Geometry check sheet. Reference: the model listing, model coordinates, mm. Face numbers are marked on the shaded views. A direction names the side the tool comes from. Give positions to 0.01 mm unless a question says otherwise; leave off trailing zeros. Write each loop counter-clockwise with the first axis right and the second up, starting at its lowest first coordinate (ties: lowest second). Pieces come first, ordered by that corner, then holes. Notation, with made-up numbers: (-2.75, 82.5) -> (21.25, 82.5) arc R11 cw to (21.25, 92.5) -> close; hole circle Ø5 at (-2, 31). An arc over 180 degrees is marked (long way). Write item = value, one per line. Start each with the question number.
1. Mould release check, pull along Y, two halves, no side actions. Record for the marked faces 1, 2 and 3: pulls with the +Y half, pulls with the -Y half, needs draft (parallel to the pull), parting line crosses it, or undercut.
2. Cross-section at A-A, the plane y = 21.5. Record the cut outline in (x, z), plus the area to 3 significant figures.
3. Cross-section at C-C, the plane x = -64. Record the cut outline in (y, z), plus the area to 3 significant figures.
4. Thickness scan on line 1 along X through (y, z) = (-19, 72); line 2 along Z through (x, y) = (-45.5, -22). Record the ranges inside material, lowest first.
5. Cross-section at B-B, the plane z = 35. Record the cut outline in (x, y).
6. Depth check by flat-ended pin: P1, Ø1.5, axis at x = -28.5, y = -27, coming from the +Z side; P2, Ø3, axis at y = 12.5, z = 93, coming from the -X side. Enter the tip coordinate at first touch or a pass-through.
7. Set-up check for the marked faces 4 and 5: record each of +Z, -Z, +X, -X, +Y, -Y from which the full face is reachable in a straight line by a thin tool's end or side.
```python
from build123d import *

# Parameters (mm, degrees)
F1_DEPTH      = 38.1
F1_DEPTH_BACK = 38.1


with BuildPart() as f1:
    # F0 (on Front) → F1 (new body, two sides)
    with BuildSketch(Plane.XZ) as f1_sk:
        Polygon((0, 0), (0, 152.4), (-25.4, 152.4), (-25.4, 25.4), (-76.2, 25.4), (-76.2, 0), align=None)
    extrude(amount=F1_DEPTH)
    extrude(f1_sk.sketch, amount=-F1_DEPTH_BACK)


solid = f1.part
```
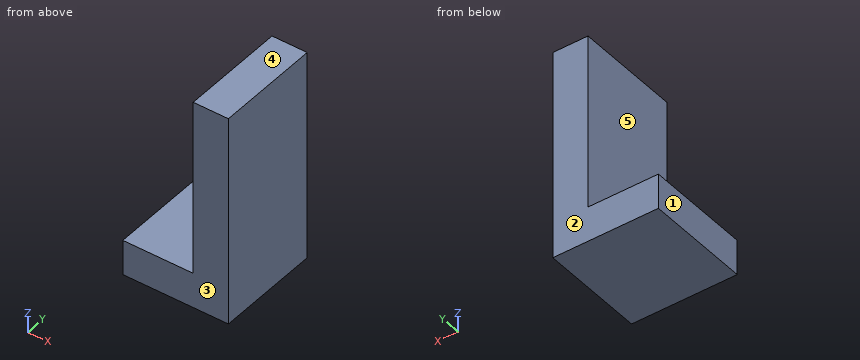
Answers:
q1.face_1 = needs draft
q1.face_2 = pulls with the +Y half
q1.face_3 = pulls with the -Y half
q2.outline = (-76.2, 0) -> (0, 0) -> (0, 152.4) -> (-25.4, 152.4) -> (-25.4, 25.4) -> (-76.2, 25.4) -> close
q2.area = 5,160 mm^2
q3.outline = (-38.1, 0) -> (38.1, 0) -> (38.1, 25.4) -> (-38.1, 25.4) -> close
q3.area = 1,940 mm^2
q4.line_1 = -25.4 to 0
q4.line_2 = 0 to 25.4
q5.outline = (-25.4, -38.1) -> (0, -38.1) -> (0, 38.1) -> (-25.4, 38.1) -> close
q6.P1 = 25.4
q6.P2 = -25.4
q7.face_4 = +Z, +X, -X, +Y, -Y
q7.face_5 = +Z, -X, +Y, -Y
